Check sheet for the modelled part. Datum: model origin and axes. Units: mm. A direction names the side the tool comes from. Round coordinates to 2 decimals unless told otherwise and drop trailing zeros. Write each loop counter-clockwise with the first axis right and the second up, starting at its lowest first coordinate (ties: lowest second). Pieces come first, ordered by that corner, then holes.
from build123d import *

# Parameters (mm, degrees)
F0_R     = 11.0625
F1_DEPTH = 11
F2_R     = 5
F3_R     = 11.0625
F4_DEPTH = 2
F6_DEPTH = 2


with BuildPart() as f1:
    # F0 (on Top) → F1 (new body)
    with BuildSketch(Plane.XY):
        Polygon((25, 14.433757), (0, 57.735027), (-25, 14.433757), align=None)
        with Locations((0, 28.867513)):
            Circle(F0_R, mode=Mode.SUBTRACT)
        Polygon((0, -28.867513), (-25, 14.433757), (-50, -28.867513), align=None)
        with Locations((-25, -14.433757)):
            Circle(F0_R, mode=Mode.SUBTRACT)
        Polygon((50, -28.867513), (25, 14.433757), (0, -28.867513), align=None)
        with Locations((25, -14.433757)):
            Circle(F0_R, mode=Mode.SUBTRACT)
        Polygon((25, 14.433757), (-25, 14.433757), (0, -28.867513), align=None)
        Circle(F0_R, mode=Mode.SUBTRACT)
    extrude(amount=F1_DEPTH)

    # F2
    f2_edges = [f1.edges().sort_by_distance(p)[0] for p in [
        (50, -28.867513, 5.5),
        (0, 57.735027, 5.5),
        (-50, -28.867513, 5.5),
    ]]
    fillet(f2_edges, radius=F2_R)

    # F3 (on face) → F4 (cut)
    with BuildSketch(Plane.XY.offset(11)):
        Polygon((-22.5, 12.990381), (0, -25.980762), (22.5, 12.990381), align=None)
        Circle(F3_R, mode=Mode.SUBTRACT)
    extrude(amount=-F4_DEPTH, mode=Mode.SUBTRACT)

    # F5 (on face) → F6 (cut)
    with BuildSketch(Plane(origin=(0, 0, 0), x_dir=(1, 0, 0), z_dir=(0, 0, -1))):
        Polygon((-22.5, -12.990381), (22.5, -12.990381), (0, 25.980762), align=None)
    extrude(amount=-F6_DEPTH, mode=Mode.SUBTRACT)


solid = f1.part
1. Release check for a two-part mould opening along X. For faces 1 (the flat face through (0, 12.99, 1)), 2 (the flat face through (0, 12.99, 10)), 3 (the cylindrical face through (-0.073, 52.734, 5.577)), 4 (the cylindrical face through (45.71, -26.3, 5.58)) record: released by +X, released by -X, zero draft, split by the parting line, or undercut.
2. Go/stop test with flat-tipped pins: pin 1 (1.5 mm diameter, centred on y = 9, z = 1.5, fed in from -X); pin 2 (1 mm diameter, centred on x = -25.5, z = 5, fed in from +Y); pin 3 (3 mm diameter, centred on y = 43.5, z = 9, fed in from -X); pin 4 (8 mm diameter, centred on x = 9.5, y = 32, fed in from +Z). Record where each tip stops, or that it passes through.
3. Sectioned sample at C-C, the plane x = 10. Enter the section's corners in (y, z).
4. Sectioned sample at B-B, the plane z = 4.75. Enter the section's corners in (x, y) (1 decimal), plus the area to 3 significant figures.
5. Sectioned sample at D-D, the plane y = 9.5. Enter the section's corners in (x, z).
6. Scan lines: line 1 along Y through (x, z) = (0, 6.75); line 2 along X through (y, z) = (-22, 10); line 3 along Y through (x, z) = (19.5, 1.5). Record each from-to range of solid material in increasing order.
7. Sectioned sample at A-A, the plane x = -26.5. Enter the section's corners in (y, z), plus the area to 3 significant figures.
8. Set-up check for faces 5 (the flat face through (-11.41, -6.22, 10.01)), 6 (the cylindrical face through (-2.4, -10.8, 5.5)), 7 (the flat face through (-11.09, -6.77, 0.99)): record each of +Z, -Z, +X, -X, +Y, -Y from which the full face is reachable in a straight line by a thin tool's end or side.
Computed values:
1. face 1: undercut
1. face 2: undercut
1. face 3: split by the parting line
1. face 4: released by +X
2. pin 1: stops at x = -28.57
2. pin 2: stops at y = 14.43
2. pin 3: stops at x = -9.08
2. pin 4: stops at z = 11
3. outline: (-28.87, 0) - (-8.66, 0) - (-8.66, 2) - (-4.73, 2) - (-4.73, 9) - (-8.66, 9) - (-8.66, 11) - (-28.87, 11) - close; (4.73, 2) - (12.99, 2) - (12.99, 0) - (24.14, 0) - (24.14, 11) - (12.99, 11) - (12.99, 9) - (4.73, 9) - close; (33.6, 0) - (40.41, 0) - (40.41, 11) - (33.6, 11) - close
4. outline: (-45.7, -21.4) arc R5 ccw to (-41.3, -28.9) - (41.3, -28.9) arc R5 ccw to (45.7, -21.4) - (4.3, 50.2) arc R5 ccw to (-4.3, 50.2) - close; hole circle Ø22.1 at (-25, -14.4); hole circle Ø22.1 at (0, 0); hole circle Ø22.1 at (0, 28.9); hole circle Ø22.1 at (25, -14.4)
4. area: 2,740 mm2
5. outline: (-27.85, 0) - (-20.48, 0) - (-20.48, 2) - (-5.67, 2) - (-5.67, 9) - (-20.48, 9) - (-20.48, 11) - (-27.85, 11) - close; (5.67, 2) - (20.48, 2) - (20.48, 0) - (27.85, 0) - (27.85, 11) - (20.48, 11) - (20.48, 9) - (5.67, 9) - close
6. line 1: y = -28.87 to -11.06, 11.06 to 17.81, 39.93 to 52.74
6. line 2: x = -45.98 to -33.07, -16.93 to -2.3, 2.3 to 16.93, 33.07 to 45.98
6. line 3: y = -28.87 to -24.03, -4.84 to 7.79, 12.99 to 23.96
7. outline: (-28.87, 0) - (-25.39, 0) - (-25.39, 11) - (-28.87, 11) - close; (-3.47, 0) - (11.84, 0) - (11.84, 11) - (-3.47, 11) - close
7. area: 207 mm2
8. face 5: +Z
8. face 6: +Z, -Z
8. face 7: -Z
